Could you check a few things on this model? Use its own coordinates, in mm. A direction names the side the tool comes from. Coordinates: 2 decimals unless noted, no trailing zeros. Loops run counter-clockwise (first coordinate to the right, second up) from the corner with the lowest first, then second, coordinate; pieces in that order, holes last. Notation, with made-up numbers: (85.25, -36.75) - (128.25, -36.75) arc R20 cw to (128.25, -3.75) - close; hole circle Ø11 at (-28, 63). An arc over 180 degrees is marked (long way). One line per item, written item: value. Start each with the question number.
(1) I'm going to push flat-ended pins straight in: P1, Ø1.9, axis at x = 3, y = 9.5, coming from the +Z side; P2, Ø5, axis at x = 11, z = 6, coming from the +Y side. Where does each tip first touch, or does it pass through?
(2) If we section it at B-B on x = 2: Write out the boundary of the cut face in (y, z), then the cut area to 3 significant figures.
(3) If we mould it in two halves opening along Z, with no side actions, what happens to faces 1 (the face through (-9.237, 14.006, 8.734)), 2 (the face through (-9.237, 2.576, 8.734)), 3 (the face through (0, 0, 0)), 4 (the face through (0, 3, 12.954))? For each: pulls with the +Z half, pulls with the -Z half, needs draft (parallel to the pull), parting line crosses it, or undercut.
(4) If we section it at A-A on z = 11: Write out the boundary of the cut face in (x, y), then the cut area to 3 significant figures.
(5) On a 3-axis mill with a long thin cutter (end or side, diameter ignored), from which of +Z, -Z, +X, -X, +Y, -Y can I reach the whole of each face in a straight line? I mean faces 5 (the face through (0, 11.43, 4)), 6 (the face through (12.099, 2.576, 8.734)). Say none if no direction works.
(6) If we section it at D-D on x = -13.5: Write out the boundary of the cut face in (y, z), then the cut area to 3 significant figures.
(7) If I drill on line 1 along X through (y, z) = (12.25, 4); line 2 along Y through (x, z) = (16, -5.25); line 3 along X through (y, z) = (15.25, 1.75), over which ranges is the centre line in solid material (lowest first)? Write a range as from..to.
(8) If we section it at C-C on z = 6.75: Write out the boundary of the cut face in (x, y).
```python
from build123d import *

# Parameters (mm, degrees)
SKETCH1_W           = 50.8
SKETCH1_H           = 25.908
BOSS_EXTRUDE1_DEPTH = 5.08
SKETCH2_W           = 50.8
SKETCH2_H           = 7.62
BOSS_EXTRUDE2_DEPTH = 6.35
SKETCH3_W           = 50.8
SKETCH3_H           = 7.62
BOSS_EXTRUDE3_DEPTH = 5.08
SKETCH4_W           = 50.8
SKETCH4_H           = 5.08
BOSS_EXTRUDE4_DEPTH = 18.288
SKETCH5_R           = 4.7625
CUT_EXTRUDE1_DEPTH  = 33.947628382


with BuildPart() as part:
    # Sketch1 → Boss-Extrude1 (new body)
    with BuildSketch(Plane(origin=(0, 0, 0), x_dir=(1, 0, 0), z_dir=(0, 1, 0))):
        Rectangle(SKETCH1_W, SKETCH1_H)
    extrude(amount=BOSS_EXTRUDE1_DEPTH)

    # Sketch2 → Boss-Extrude2 (add)
    with BuildSketch(Plane(origin=(0, 5.08, 0), x_dir=(1, 0, 0), z_dir=(0, 1, 0))):
        with Locations((0, 9.144)):
            Rectangle(SKETCH2_W, SKETCH2_H)
    extrude(amount=BOSS_EXTRUDE2_DEPTH)

    # Sketch3 → Boss-Extrude3 (add)
    with BuildSketch(Plane(origin=(0, 11.43, 0), x_dir=(1, 0, 0), z_dir=(0, 1, 0))):
        with Locations((0, 9.144)):
            Rectangle(SKETCH3_W, SKETCH3_H)
    extrude(amount=BOSS_EXTRUDE3_DEPTH)

    # Sketch4 → Boss-Extrude4 (add)
    with BuildSketch(Plane.XY.offset(-5.334)):
        with Locations((0, 13.97)):
            Rectangle(SKETCH4_W, SKETCH4_H)
    extrude(amount=BOSS_EXTRUDE4_DEPTH)

    # Sketch5 → Cut-Extrude1 (cut, through all)
    with BuildSketch(Plane(origin=(0, 16.51, 0), x_dir=(1, 0, 0), z_dir=(0, 1, 0))):
        with Locations(Location((-10.668, -4.191, 0), (0, 0, 270))):
            Circle(SKETCH5_R)
        with Locations(Location((10.668, -4.191, 0), (0, 0, 270))):
            Circle(SKETCH5_R)
    extrude(amount=-CUT_EXTRUDE1_DEPTH, mode=Mode.SUBTRACT)


solid = part.part
```
Values:
1. P1: stops at z = -5.33
1. P2: passes through
2. outline: (0, -12.95) - (16.51, -12.95) - (16.51, 12.95) - (11.43, 12.95) - (11.43, -5.33) - (5.08, -5.33) - (5.08, 12.95) - (0, 12.95) - close
2. area: 312 mm2
3. face 1: undercut
3. face 2: undercut
3. face 3: needs draft
3. face 4: pulls with the +Z half
4. outline: (-25.4, 0) - (25.4, 0) - (25.4, 5.08) - (-25.4, 5.08) - close; (-25.4, 11.43) - (25.4, 11.43) - (25.4, 16.51) - (-25.4, 16.51) - close
4. area: 516 mm2
5. face 5: +Z, +X, -X
5. face 6: +Y, -Y
6. outline: (0, -12.95) - (16.51, -12.95) - (16.51, 0.36) - (11.43, 0.36) - (11.43, -5.33) - (5.08, -5.33) - (5.08, 0.36) - (0, 0.36) - close; (0, 8.02) - (5.08, 8.02) - (5.08, 12.95) - (0, 12.95) - close; (11.43, 8.02) - (16.51, 8.02) - (16.51, 12.95) - (11.43, 12.95) - close
6. area: 234 mm2
7. line 1: x = -25.4..-15.43, -5.91..5.91, 15.43..25.4
7. line 2: y = 0..5.08, 11.43..16.51
7. line 3: x = -25.4..-14.76, -6.58..6.58, 14.76..25.4
8. outline: (-25.4, 0) - (-14.68, 0) - (-14.68, 5.08) - (-25.4, 5.08) - close; (-25.4, 11.43) - (-14.68, 11.43) - (-14.68, 16.51) - (-25.4, 16.51) - close; (-6.65, 0) - (6.65, 0) - (6.65, 5.08) - (-6.65, 5.08) - close; (-6.65, 11.43) - (6.65, 11.43) - (6.65, 16.51) - (-6.65, 16.51) - close; (14.68, 0) - (25.4, 0) - (25.4, 5.08) - (14.68, 5.08) - close; (14.68, 11.43) - (25.4, 11.43) - (25.4, 16.51) - (14.68, 16.51) - close
